from build123d import *

# Parameters (mm, degrees)
F0_W     = 127
F0_H     = 76.2
F1_DEPTH = 12.7
F2_R     = 6.35
F3_DEPTH = 12.701
F4_W     = 12.7
F4_H     = 50.8
F6_W     = 9.855053
F6_H     = 6.35
F8_R     = 5.08
F9_SIZE  = 5.08


with BuildPart() as f1:
    # F0 (on Top) → F1 (new body)
    with BuildSketch(Plane.XY):
        Rectangle(F0_W, F0_H)
    extrude(amount=F1_DEPTH)

    # F2 (on face) → F3 (cut, through all)
    with BuildSketch(Plane.XY.offset(12.7)):
        with Locations((-50.8, 25.4)):
            Circle(F2_R)
        with Locations((50.8, 25.4)):
            Circle(F2_R)
        with Locations((-50.8, -25.4)):
            Circle(F2_R)
        with Locations((50.8, -25.4)):
            Circle(F2_R)
    extrude(amount=-F3_DEPTH, mode=Mode.SUBTRACT)

    # F4 (on Right) → F5 (revolve)
    with BuildSketch(Plane.YZ):
        with Locations((6.35, 38.1)):
            Rectangle(F4_W, F4_H)
    revolve(axis=Axis((0, 0, 38.1), (0, 0, 1)))

    # F6 (on Front) → F7 (revolve, cut)
    with BuildSketch(Plane.XZ):
        with Locations((15.087526, 41.275)):
            Rectangle(F6_W, F6_H)
    revolve(axis=Axis((0, 0, 12.7), (0, 0, 1)), mode=Mode.SUBTRACT)

    # F8
    f8_edges = [f1.edges().sort_by_distance(p)[0] for p in [
        (0, -12.7, 12.7),
        (0, -12.7, 63.5),
    ]]
    fillet(f8_edges, radius=F8_R)

    # F9
    f9_edges = [f1.edges().sort_by_distance(p)[0] for p in [
        (-63.5, 0, 12.7),
        (0, -38.1, 12.7),
        (63.5, 0, 12.7),
        (0, 38.1, 12.7),
    ]]
    chamfer(f9_edges, length=F9_SIZE)


solid = f1.part
Source: CAD feature listing. Evaluate the final solid. Frame: model axes, mm. A direction names the side the tool comes from. Coordinates: 2 decimals unless noted, no trailing zeros. Loops run counter-clockwise (first coordinate to the right, second up) from the corner with the lowest first, then second, coordinate; pieces in that order, holes last. Notation, with made-up numbers: (43, 72.25) - (78, 72.25) arc R17 ccw to (78, 77.25) - close; hole circle Ø1 at (-39, 18.5). An arc over 180 degrees is marked (long way). Return JSON: item names as keys, results as strings.
Q1. Section C-C, the plane x = 0. Return loops of the section in (y, z).
Results:
{"outline": "(-38.1, 0) - (38.1, 0) - (38.1, 7.62) - (33.02, 12.7) - (17.78, 12.7) arc R5.08 cw to (12.7, 17.78) - (12.7, 38.1) - (10.16, 38.1) - (10.16, 44.45) - (12.7, 44.45) - (12.7, 58.42) arc R5.08 ccw to (7.62, 63.5) - (-7.62, 63.5) arc R5.08 ccw to (-12.7, 58.42) - (-12.7, 44.45) - (-10.16, 44.45) - (-10.16, 38.1) - (-12.7, 38.1) - (-12.7, 17.78) arc R5.08 cw to (-17.78, 12.7) - (-33.02, 12.7) - (-38.1, 7.62) - close"}
Q2. Section B-B, the plane x = 50.8. Return loops of the section in (y, z), plus the area to 3 significant figures.
Results:
{"outline": "(-38.1, 0) - (-31.75, 0) - (-31.75, 12.7) - (-33.02, 12.7) - (-38.1, 7.62) - close; (-19.05, 0) - (19.05, 0) - (19.05, 12.7) - (-19.05, 12.7) - close; (31.75, 0) - (38.1, 0) - (38.1, 7.62) - (33.02, 12.7) - (31.75, 12.7) - close", "area": "619 mm2"}
Q3. Contact query for flat-ended pins moving along their axis: P1, Ø8, axis at x = -19, y = 19.5, coming from the -Z side; P2, Ø8, axis at y = -11.5, z = 23, coming from the +X side; P3, Ø1, axis at x = 8, z = 17.5, coming from the +Y side; P4, Ø10, axis at x = 33, y = -8, coming from the +Z side. Output: stop coordinate, or through.
Results:
{"P1": "z = 0", "P2": "x = 10.25", "P3": "y = 10.26", "P4": "z = 12.7"}
Q4. Mould query, pull axis Z, two halves, no side actions, for faces 1 (the flat face through (6, 9, 44.45)), 2 (the cylindrical face through (56.666, -27.832, 6.439)), 3 (the flat face through (61, -0.53, 10.12)). Classes: released by +Z, released by -Z, zero draft, split by the parting line, or undercut.
Results:
{"face 1": "undercut", "face 2": "zero draft", "face 3": "released by +Z"}
Q5. Access query for faces 4 (the cylindrical face through (12.4, -2.75, 51.53)), 5 (the cylindrical face through (-2.2, -9.92, 41.32)), 6 (the cylindrical face through (56.666, 22.968, 6.439)). Directions: +Z, -Z, +X, -X, +Y, -Y. A direction counts if a zero-diameter tool reaches every point of the face in a straight line with its end or side. Return the directions, or none.
Results:
{"face 4": "+Z", "face 5": "none", "face 6": "+Z, -Z"}
Q6. Section A-A, the plane y = -25.4. Return loops of the section in (x, z), plus the area to 3 significant figures.
Results:
{"outline": "(-63.5, 0) - (-57.15, 0) - (-57.15, 12.7) - (-58.42, 12.7) - (-63.5, 7.62) - close; (-44.45, 0) - (44.45, 0) - (44.45, 12.7) - (-44.45, 12.7) - close; (57.15, 0) - (63.5, 0) - (63.5, 7.62) - (58.42, 12.7) - (57.15, 12.7) - close", "area": "1,260 mm2"}
Q7. Material intervals for line 1 along Y through (x, z) = (50.8, 5.25); line 2 along X through (y, z) = (-25, 3); line 3 along Z through (x, y) = (-9, 26), sorted ascending.
Results:
{"line 1": "-38.1 to -31.75, -19.05 to 19.05, 31.75 to 38.1", "line 2": "-63.5 to -57.14, -44.46 to 44.46, 57.14 to 63.5", "line 3": "0 to 12.7"}
Q8. Section D-D, the plane z = 42. Return loops of the section in (x, y), plus the area to 3 significant figures.
Results:
{"outline": "circle Ø20.32 at (0, 0)", "area": "324 mm2"}
